Autodesk Inventor part; units mm, degrees
ref_plane "YZ Plane" through (0, 0, 0) normal (1, 0, 0) x (0, 1, 0)
ref_plane "XZ Plane" through (0, 0, 0) normal (0, 1, 0) x (-1, 0, 0)
ref_plane "XY Plane" through (0, 0, 0) normal (0, 0, 1) x (1, 0, 0)
sketch "Sketch1" plane through (0, 0, 0) normal (0, 0, 1) x (1, 0, 0)
  line L0 (2.35, 1.3568) -> (2.35, -1.3568)
  line L1 (2.35, -1.3568) -> (0, -2.7135)
  line L2 (0, -2.7135) -> (-2.35, -1.3568)
  line L3 (-2.35, 1.3568) -> (-2.35, -1.3568)
  line L4 (-2.35, 1.3568) -> (0, 2.7135)
  line L5 (0, 2.7135) -> (2.35, 1.3568)
  circle A0 centre (0, 0) radius 2.7135 construction
  line L6 (0, 29.0365) -> (0, -7.2493) construction
  line L7 (0, -14.5064) -> (0, 36.2936)
  line L8 (-3.799, 0) -> (3.799, 0)
  dimension "d0" = 5.4271
  dimension "d20" = 4.7
  dimension "d21" = 2.7136
extrude "Hexagon1" add sketch "Sketch1" along normal blind 5
hole "Hole1" at (0, 0, 0) direction (0, 0, 1) diameter 2.459 depth 4.5
sketch "Sketch2" plane through (0, 0, 5) normal (0, 0, 1) x (1, 0, 0)
  circle A0 centre (0, 0) radius 1.4
  dimension "d22" = 2.8
extrude "Extrusion2" add sketch "Sketch2" along normal blind 4
thread "Thread3"
properties part number "Spacer-M3-05" material "Brass, Soft Yellow, Welded"
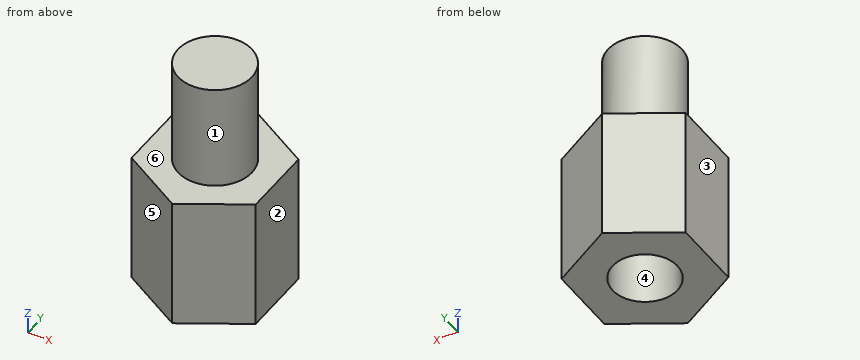
For this review, take the finished solid that the model builds, in its own axes (mm). Face numbers are marked on the shaded views. A direction names the side the tool comes from. Round coordinates to 2 decimals unless told otherwise and drop trailing zeros. Order: outer loops, then holes, each group sorted by start corner. A loop starts at its lowest first (then second) coordinate and runs counter-clockwise, first axis right, second up. Notation, with made-up numbers: (53, 76) -> (88, 76) arc R22 cw to (88, 114) -> close; hole circle Ø5 at (2.5, 40). An arc over 180 degrees is marked (long way). Write item = value, one per line. Start each with the question number.
1) Tool access review of the marked faces 5 and 6: name each direction out of +Z, -Z, +X, -X, +Y, -Y from which nothing blocks a thin tool from reaching the whole face with its end or side.
2) Take a section at C-C on x = 0.6. State the section outline as (y, z) points.
3) To check wall thickness, follow line 1 (X direction, y = 0, z = 2.25); line 2 (Z direction, x = -1.1, y = 1.25); line 3 (Y direction, x = -0.5, z = 1.75). State the ranges of each line that lie inside material, in increasing order. Write a range as from..to.
4) Take a section at B-B on y = 0. State the section outline as (x, z) points.
5) Take a section at D-D on z = 7.25. State the section outline as (x, y) points.
6) The part is to be moulded in two halves that separate along X. For the marked faces 1, 2, 3 and 4, say which applies: +X half, -X half, draft (parallel to the pull), parting line (faces both ways), or undercut.
7) Take a section at A-A on z = 1.75. State the section outline as (x, y) points.
8) Insertion check: pin 1 (1.5 mm diameter, centred on x = -0.5, z = 3.5, fed in from -Y); pin 2 (0.7 mm diameter, centred on x = 0, y = 0, fed in from -Z). Each pin has a flat end and moves straight along its axis. Give the tip position at first contact, or say it passes through.
Verdict:
q1.face_5 = +Z, -Z, -X, -Y
q1.face_6 = +Z
q2.outline = (-2.37, 0) -> (-1.07, 0) -> (-1.07, 4.5) -> (1.07, 4.5) -> (1.07, 0) -> (2.37, 0) -> (2.37, 5) -> (1.26, 5) -> (1.26, 9) -> (-1.26, 9) -> (-1.26, 5) -> (-2.37, 5) -> close
q3.line_1 = -2.35..-1.23, 1.23..2.35
q3.line_2 = 0..5
q3.line_3 = -2.42..-1.12, 1.12..2.42
q4.outline = (-2.35, 0) -> (-1.23, 0) -> (-1.23, 4.5) -> (1.23, 4.5) -> (1.23, 0) -> (2.35, 0) -> (2.35, 5) -> (1.4, 5) -> (1.4, 9) -> (-1.4, 9) -> (-1.4, 5) -> (-2.35, 5) -> close
q5.outline = circle Ø2.8 at (0, 0)
q6.face_1 = parting line
q6.face_2 = +X half
q6.face_3 = -X half
q6.face_4 = undercut
q7.outline = (-2.35, -1.36) -> (0, -2.71) -> (2.35, -1.36) -> (2.35, 1.36) -> (0, 2.71) -> (-2.35, 1.36) -> close; hole circle Ø2.46 at (0, 0)
q8.pin_1 = -2.71
q8.pin_2 = 4.5
